from build123d import *

# Parameters (mm, degrees)
SKETCH_1_R      = 40
SKETCH_1_R_2    = 10
EXTRUDE_1_DEPTH = 10
SKETCH_2_W      = 9.777839157
SKETCH_2_H      = 8.649626946
EXTRUDE_2_DEPTH = 10


with BuildPart() as part:
    # 草图1 → 凸台-拉伸1 (new body)
    with BuildSketch(Plane(origin=(0, 0, 0), x_dir=(0, 0, -1), z_dir=(1, 0, 0))):
        Circle(SKETCH_1_R)
        Circle(SKETCH_1_R_2, mode=Mode.SUBTRACT)
    extrude(amount=EXTRUDE_1_DEPTH)

    # 草图2 → 凸台-拉伸2 (add)
    with BuildSketch(Plane(origin=(10, 0, 0), x_dir=(0, 0, -1), z_dir=(1, 0, 0))):
        with Locations((24.181348377, 0)):
            Rectangle(SKETCH_2_W, SKETCH_2_H)
    extrude(amount=EXTRUDE_2_DEPTH)


solid = part.part
Work out the finished part from the listing and answer in its coordinate system (mm). A direction names the side the tool comes from. Round coordinates to 2 decimals unless told otherwise and drop trailing zeros. Write each loop counter-clockwise with the first axis right and the second up, starting at its lowest first coordinate (ties: lowest second). Pieces come first, ordered by that corner, then holes. Notation, with made-up numbers: (-16.75, -29) - (28.25, -29) arc R20 ccw to (28.25, 8) - close; hole circle Ø7 at (-14, -4). An arc over 180 degrees is marked (long way). Answer in a Markdown table with one row per item. Add a question column.
1. Given pin 1 (6 mm diameter, centred on x = 11, z = 25.5, fed in from -Y); pin 2 (7 mm diameter, centred on x = 17, y = -0.5, fed in from -Z); pin 3 (3 mm diameter, centred on x = 17, z = -24, fed in from +Y); pin 4 (12 mm diameter, centred on y = 28, z = -31.5, fed in from -X), each flat-ended and moving along its own axis, determine where each tip first touches the part or whether it passes through.
2. A cutting plane is placed at C-C, the plane x = 6.75. Determine the outline of the cut face in (y, z), and give its area (3 significant figures).
3. Find the intervals of material crossed by line 1 along Y through (x, z) = (4.75, 0); line 2 along X through (y, z) = (-19.5, 8); line 3 along Z through (x, y) = (4, -3.5), in increasing order. Write a range as from..to.
4. The mould has two halves that part along Z. Classify faces 1 (the cylindrical face through (4.93, -39.05, 8.67)), 2 (the cylindrical face through (4.93, -9.76, 2.17)), 3 (the flat face through (15, -4.325, -24)): +Z half, -Z half, draft (parallel to the pull), parting line (faces both ways), or undercut.
5. A cutting plane is placed at A-A, the plane z = 0. Determine the outline of the cut face in (x, y).
6. A cutting plane is placed at B-B, the plane y = 0. Determine the outline of the cut face in (x, z), and give its area (3 significant figures).
7. A cutting plane is placed at D-D, the plane y = -34. Determine the outline of the cut face in (x, z).
8. For faces 4 (the flat face through (15, 0, -19.292)), 5 (the flat face through (0, -8, -8)), 6 (the flat face through (15, 0, -29.07)), 7 (the flat face through (15, 4.325, -24)), determine the directions among +Z, -Z, +X, -X, +Y, -Y from which every point of the face is accessible in a straight line to the end or side of a thin tool.
Worked out:
| question | item | result |
|---|---|---|
| 1 | pin 1 | y = -32.95 |
| 1 | pin 2 | z = -29.07 |
| 1 | pin 3 | y = 4.32 |
| 1 | pin 4 | x = 0 |
| 2 | outline | circle Ø80 at (0, 0); hole circle Ø20 at (0, 0) |
| 2 | area | 4,710 mm^2 |
| 3 | line 1 | -40..-10, 10..40 |
| 3 | line 2 | 0..10 |
| 3 | line 3 | -39.85..-9.37, 9.37..39.85 |
| 4 | face 1 | parting line |
| 4 | face 2 | undercut |
| 4 | face 3 | draft |
| 5 | outline | (0, -40) - (10, -40) - (10, -10) - (0, -10) - close; (0, 10) - (10, 10) - (10, 40) - (0, 40) - close |
| 6 | outline | (0, -40) - (10, -40) - (10, -29.07) - (20, -29.07) - (20, -19.29) - (10, -19.29) - (10, -10) - (0, -10) - close; (0, 10) - (10, 10) - (10, 40) - (0, 40) - close |
| 6 | area | 698 mm^2 |
| 7 | outline | (0, -21.07) - (10, -21.07) - (10, 21.07) - (0, 21.07) - close |
| 8 | face 4 | +Z, +X, +Y, -Y |
| 8 | face 5 | +Z, -Z, -X, +Y, -Y |
| 8 | face 6 | -Z, +X, +Y, -Y |
| 8 | face 7 | +Z, -Z, +X, +Y |
